Work out the finished part from the listing and answer in its coordinate system (mm). Round coordinates to 2 decimals unless told otherwise and drop trailing zeros. Loops run counter-clockwise (first coordinate to the right, second up) from the corner with the lowest first, then second, coordinate; pieces in that order, holes last.
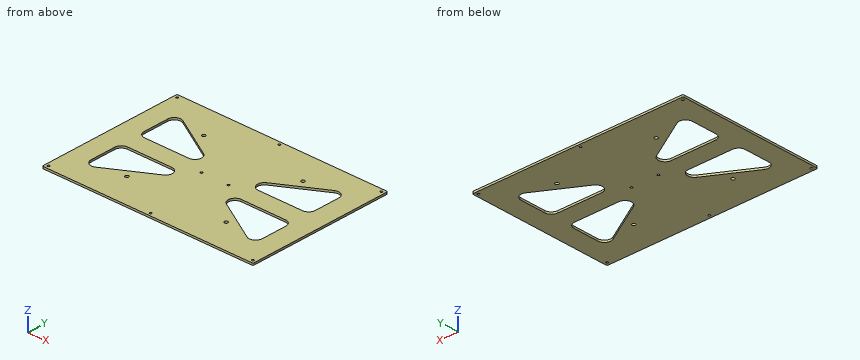
```python
from build123d import *

# Parameters (mm, degrees)
F0_R     = 1.7
F1_DEPTH = 3
F3_DEPTH = 3.001
F4_R     = 2.6
F5_DEPTH = 25


with BuildPart() as f1:
    # F0 (on Top) → F1 (new body)
    with BuildSketch(Plane.XY):
        with BuildLine():
            Line((-157.5, -109.5), (157.5, -109.5))
            ThreePointArc((157.5, -109.5), (158.914214, -108.914214), (159.5, -107.5))
            Line((159.5, -107.5), (159.5, 107.5))
            ThreePointArc((159.5, 107.5), (158.914214, 108.914214), (157.5, 109.5))
            Line((157.5, 109.5), (-157.5, 109.5))
            ThreePointArc((-157.5, 109.5), (-158.914214, 108.914214), (-159.5, 107.5))
            Line((-159.5, 107.5), (-159.5, -107.5))
            ThreePointArc((-159.5, -107.5), (-158.914214, -108.914214), (-157.5, -109.5))
        make_face()
        with Locations((-154.5, -104.5)):
            Circle(F0_R, mode=Mode.SUBTRACT)
        with Locations((0, -104.5)):
            Circle(F0_R, mode=Mode.SUBTRACT)
        with Locations((154.5, -104.5)):
            Circle(F0_R, mode=Mode.SUBTRACT)
        with Locations((-20.5, 0)):
            Circle(F0_R, mode=Mode.SUBTRACT)
        with Locations((-154.5, 104.5)):
            Circle(F0_R, mode=Mode.SUBTRACT)
        with Locations((20.5, 0)):
            Circle(F0_R, mode=Mode.SUBTRACT)
        with Locations((0, 104.5)):
            Circle(F0_R, mode=Mode.SUBTRACT)
        with Locations((154.5, 104.5)):
            Circle(F0_R, mode=Mode.SUBTRACT)
    extrude(amount=F1_DEPTH)

    # F2 (on face) → F3 (cut, through all)
    with BuildSketch(Plane.XY.offset(3)):
        with BuildLine():
            Line((-129.5, 62.243366), (-129.5, 23.88142))
            ThreePointArc((-129.5, 23.88142), (-126.571068, 16.810352), (-119.5, 13.88142))
            Line((-119.5, 13.88142), (-52.560989, 13.88142))
            ThreePointArc((-52.560989, 13.88142), (-42.897598, 21.3087), (-47.588749, 32.557642))
            Line((-47.588749, 32.557642), (-114.527761, 70.919589))
            ThreePointArc((-114.527761, 70.919589), (-124.513861, 70.895603), (-129.5, 62.243366))
        make_face()
        with BuildLine():
            Line((52.560989, 13.88142), (119.5, 13.88142))
            ThreePointArc((119.5, 13.88142), (126.571068, 16.810352), (129.5, 23.88142))
            Line((129.5, 23.88142), (129.5, 62.243366))
            ThreePointArc((129.5, 62.243366), (124.513861, 70.895603), (114.527761, 70.919589))
            Line((114.527761, 70.919589), (47.588749, 32.557642))
            ThreePointArc((47.588749, 32.557642), (42.897598, 21.3087), (52.560989, 13.88142))
        make_face()
        with BuildLine():
            ThreePointArc((114.527761, -70.919589), (124.513861, -70.895603), (129.5, -62.243366))
            Line((129.5, -62.243366), (129.5, -23.88142))
            ThreePointArc((129.5, -23.88142), (126.571068, -16.810352), (119.5, -13.88142))
            Line((119.5, -13.88142), (52.560989, -13.88142))
            ThreePointArc((52.560989, -13.88142), (42.897598, -21.3087), (47.588749, -32.557642))
            Line((47.588749, -32.557642), (114.527761, -70.919589))
        make_face()
        with BuildLine():
            Line((-129.5, -23.88142), (-129.5, -62.243366))
            ThreePointArc((-129.5, -62.243366), (-124.513861, -70.895603), (-114.527761, -70.919589))
            Line((-114.527761, -70.919589), (-47.588749, -32.557642))
            ThreePointArc((-47.588749, -32.557642), (-42.897598, -21.3087), (-52.560989, -13.88142))
            Line((-52.560989, -13.88142), (-119.5, -13.88142))
            ThreePointArc((-119.5, -13.88142), (-126.571068, -16.810352), (-129.5, -23.88142))
        make_face()
    extrude(amount=-F3_DEPTH, mode=Mode.SUBTRACT)

    # F4 (on face) → F5 (cut)
    with BuildSketch(Plane.XY.offset(3)):
        with Locations((-75, 62.5)):
            Circle(F4_R)
        with Locations((-75, -62.5)):
            Circle(F4_R)
        with Locations((75, 62.5)):
            Circle(F4_R)
        with Locations((75, -62.5)):
            Circle(F4_R)
    extrude(amount=-F5_DEPTH, mode=Mode.SUBTRACT)


solid = f1.part
```
1. Find section C-C (y = 44). Write down the section's boundary in (x, z), then the cut area to 3 significant figures.
Answer key:
outline: (-159.5, 0) - (-129.5, 0) - (-129.5, 3) - (-159.5, 3) - close; (-67.55, 0) - (67.55, 0) - (67.55, 3) - (-67.55, 3) - close; (129.5, 0) - (159.5, 0) - (159.5, 3) - (129.5, 3) - close
area: 585 mm2
2. Find section B-B (z = 1.4). Give the number of separate pieces and of enclosed holes in the cut face, then the cut area to 3 significant figures.
Answer key:
separate pieces: 1
enclosed holes: 16
area: 56,000 mm2
3. Consider probe 1 along X at (y, z) = (-104.5, 1.65); probe 2 along Y at (x, z) = (154.5, 2.25); probe 3 along Y at (x, z) = (75, 1.8). Determine where each line is inside the solid, lowest interval first.
Answer key:
probe 1: x = -159.5 to -156.2, -152.8 to -1.7, 1.7 to 152.8, 156.2 to 159.5
probe 2: y = -109.5 to -106.2, -102.8 to 102.8, 106.2 to 109.5
probe 3: y = -109.5 to -65.1, -59.9 to -48.27, -13.88 to 13.88, 48.27 to 59.9, 65.1 to 109.5
4. Find section A-A (y = -44.5). Write down the section's boundary in (x, z).
Answer key:
outline: (-159.5, 0) - (-129.5, 0) - (-129.5, 3) - (-159.5, 3) - close; (-68.43, 0) - (68.43, 0) - (68.43, 3) - (-68.43, 3) - close; (129.5, 0) - (159.5, 0) - (159.5, 3) - (129.5, 3) - close
